Model file for the job. Use its own axes, mm. Face numbers are marked on the shaded views. A direction names the side the tool comes from. Round coordinates to 2 decimals unless told otherwise and drop trailing zeros. One line per item, written item: value.
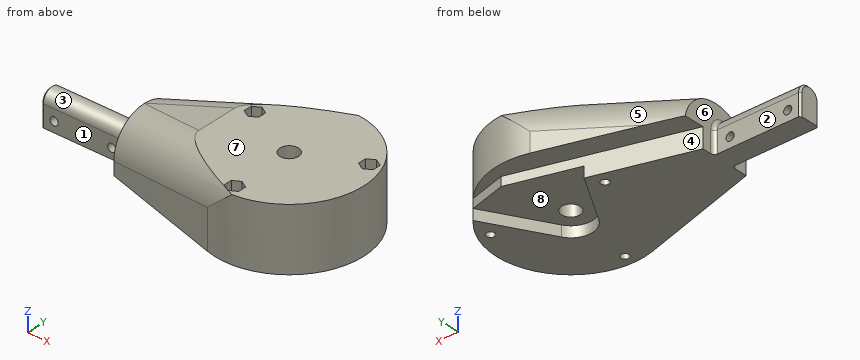
from build123d import *

# Parameters (mm, degrees)
RESSALTO_EXTRUS_O1_DEPTH = 35
CHANFRO1_SIZE            = 40
CHANFRO1_SIZE2           = 8.502262467
FILETE2_R                = 20
CORTE_EXTRUS_O2_DEPTH    = 6
CORTE_EXTRUS_O3_DEPTH    = 11
CHANFRO2_SIZE            = 10
RESSALTO_EXTRUS_O2_DEPTH = 48
CHANFRO3_SIZE            = 1
FILETE3_R                = 2
ESBO_O9_R                = 2.25
CORTE_EXTRUS_O4_DEPTH    = 342.284989024
ESBO_O10_R               = 5.15
CORTE_EXTRUS_O5_DEPTH    = 367.917618461
CORTE_EXTRUS_O7_DEPTH    = 10
ESBO_O13_R               = 2.25
CORTE_EXTRUS_O8_DEPTH    = 367.09908322


with BuildPart() as part:
    # Esboço1 → Ressalto-extrusão1 (new body)
    with BuildSketch(Plane.XY):
        with BuildLine():
            Line((-288.88140452, 80), (-220.127979697, 60.449355997))
            ThreePointArc((-220.127979697, 60.449355997), (-167.76280904, 100), (-220.127979697, 139.550644003))
            Line((-220.127979697, 139.550644003), (-288.88140452, 119.635273108))
            Line((-288.88140452, 119.635273108), (-288.88140452, 80))
        make_face()
    extrude(amount=RESSALTO_EXTRUS_O1_DEPTH)

    # Chanfro1
    chanfro1_edges = [part.edges().sort_by_distance(p)[0] for p in [
        (-288.88140452, 99.817636554, 35),
    ]]
    chanfro1_side = [part.faces().sort_by_distance(p)[0] for p in [
        (-225.798931966, 99.956743446, 35),
    ]]
    chamfer(chanfro1_edges, length=CHANFRO1_SIZE, length2=CHANFRO1_SIZE2, reference=chanfro1_side[0])

    # Filete2
    # the kernel refuses this fillet: 20 mm, written as the material it takes off along each edge
    with BuildSketch(Plane(origin=(-115.658970437, 169.81152296, 63.317302526), x_dir=(0.19213899287120792, 0.055655690116350805, -0.9797882687479528), z_dir=(-0.9411018224853822, -0.27260302876307696, -0.2000373675688854))) as filete2_piece_1:
        with BuildLine():
            CenterArc((FILETE2_R * 0.943733759019, FILETE2_R), FILETE2_R, 183.31621355, 86.68378645)
            Line((-FILETE2_R * 0.054591728164, FILETE2_R * 0.942153464743), (0, 0))
            Line((0, 0), (FILETE2_R * 0.943733759019, 0))
        make_face()
    extrude(amount=231.2501229, mode=Mode.SUBTRACT)
    with BuildSketch(Plane(origin=(-115.347800558, 30.654185994, 63.383443726), x_dir=(0.2621163849534368, 0.9634266390424966, 0.05571455754307817), z_dir=(-0.9423734554624519, 0.2679722209171675, -0.2003076615021976))) as filete2_piece_2:
        with BuildLine():
            CenterArc((FILETE2_R * 0.9446616108, FILETE2_R), FILETE2_R, 183.260002361, 86.739997639)
            Line((-FILETE2_R * 0.0537201474496, FILETE2_R * 0.943132919942), (0, 0))
            Line((0, 0), (FILETE2_R * 0.9446616108, 0))
        make_face()
    extrude(amount=231.378339467, mode=Mode.SUBTRACT)

    # Esboço6 → Corte-extrusão2 (cut)
    with BuildSketch(Plane(origin=(0, 0, 0), x_dir=(-1, 0, 0), z_dir=(0, 0, -1))):
        with BuildLine():
            Line((219.273709365, 94), (245.2234198, 138.946216915))
            Line((245.2234198, 138.946216915), (172.539389239, 138.946216915))
            Line((172.539389239, 138.946216915), (198.489099675, 94))
            ThreePointArc((198.489099675, 94), (208.88140452, 88), (219.273709365, 94))
        make_face()
    extrude(amount=-CORTE_EXTRUS_O2_DEPTH, mode=Mode.SUBTRACT)

    # Esboço7 → Corte-extrusão3 (cut)
    with BuildSketch(Plane(origin=(0, 0, 0), x_dir=(-1, 0, 0), z_dir=(0, 0, -1))):
        Polygon((179.171530951, 139.11313265), (295.618088129, 106.000524942), (295.618088129, 136.423544796), (188.948158446, 165.308096575), align=None)
    extrude(amount=-CORTE_EXTRUS_O3_DEPTH, mode=Mode.SUBTRACT)

    # Chanfro2
    # the kernel refuses this chamfer: 22.612495948, 10 mm, written as the material it takes off along each edge
    with BuildSketch(Plane(origin=(-189.392572811, 136.206689062, 11), x_dir=(0.7913619734687217, -0.6113478771924299, 0), z_dir=(0, 0, -1))) as chanfro2_piece_1:
        with BuildLine():
            Line((13.424324353, 0), (-CHANFRO2_SIZE * 0.593972278099, CHANFRO2_SIZE * 0.804485508167))
            Line((-CHANFRO2_SIZE * 0.593972278099, CHANFRO2_SIZE * 0.804485508167), (0, 0))
            ThreePointArc((0, 0), (7.133656498, -0.549382314), (13.424324353, 0))
        make_face()
    extrude(amount=40.659571502, mode=Mode.SUBTRACT)

    # Esboço8 → Ressalto-extrusão2 (add)
    with BuildSketch(Plane.ZY.offset(288.88140452)):
        with BuildLine():
            Line((0, 100.85), (12, 100.85))
            ThreePointArc((12, 100.85), (17.85, 95), (12, 89.15))
            Line((12, 89.15), (0, 89.15))
            Line((0, 89.15), (0, 100.85))
        make_face()
    extrude(amount=RESSALTO_EXTRUS_O2_DEPTH)

    # Chanfro3
    chanfro3_edges = [part.edges().sort_by_distance(p)[0] for p in [
        (-336.88140452, 89.15, 6),
        (-336.88140452, 95, 17.85),
        (-336.88140452, 100.85, 6),
    ]]
    chamfer(chanfro3_edges, length=CHANFRO3_SIZE)

    # Filete3
    filete3_edges = [part.edges().sort_by_distance(p)[0] for p in [
        (-288.88140452, 89.15, 6),
        (-288.88140452, 95, 17.85),
        (-288.88140452, 100.85, 6),
    ]]
    fillet(filete3_edges, radius=FILETE3_R)

    # Esboço9 → Corte-extrusão4 (cut, through all)
    with BuildSketch(Plane(origin=(0, 100.85, 0), x_dir=(1, 0, 0), z_dir=(0, 1, 0))):
        with Locations(Location((-329.846296891, -5.75110431, 0), (0, 0, 270))):
            Circle(ESBO_O9_R)
        with Locations(Location((-297.910035946, -5.75110431, 0), (0, 0, 270))):
            Circle(ESBO_O9_R)
    extrude(amount=-CORTE_EXTRUS_O4_DEPTH, mode=Mode.SUBTRACT)

    # Esboço10 → Corte-extrusão5 (cut, through all)
    with BuildSketch(Plane(origin=(0, 0, 0), x_dir=(-1, 0, 0), z_dir=(0, 0, -1))):
        with Locations((208.88140452, 100)):
            Circle(ESBO_O10_R)
    extrude(amount=-CORTE_EXTRUS_O5_DEPTH, mode=Mode.SUBTRACT)

    # Esboço12 → Corte-extrusão7 (cut)
    with BuildSketch(Plane.XY.offset(35)):
        Polygon((-240.599798192, 119.415541755), (-244.599798192, 117.106140678), (-244.599798192, 112.487338525), (-240.599798192, 110.177937448), (-236.599798192, 112.487338525), (-236.599798192, 117.106140678), align=None)
        Polygon((-208.88140452, 69.618802154), (-212.88140452, 67.309401077), (-212.88140452, 62.690598923), (-208.88140452, 60.381197846), (-204.88140452, 62.690598923), (-204.88140452, 67.309401077), align=None)
        Polygon((-177.163010847, 119.415541755), (-181.163010847, 117.106140678), (-181.163010847, 112.487338525), (-177.163010847, 110.177937448), (-173.163010847, 112.487338525), (-173.163010847, 117.106140678), align=None)
    extrude(amount=-CORTE_EXTRUS_O7_DEPTH, mode=Mode.SUBTRACT)

    # Esboço13 → Corte-extrusão8 (cut, through all)
    with BuildSketch(Plane.XY.offset(25)):
        with Locations((-177.163010847, 114.796739602)):
            Circle(ESBO_O13_R)
        with Locations((-208.88140452, 65)):
            Circle(ESBO_O13_R)
        with Locations((-240.599798192, 114.796739602)):
            Circle(ESBO_O13_R)
    extrude(amount=-CORTE_EXTRUS_O8_DEPTH, mode=Mode.SUBTRACT)


solid = part.part
1. Wall check: probe 1 along Z at (x, y) = (-248.5, 86); probe 2 along Y at (x, z) = (-314, 10); probe 3 along X at (y, z) = (102.5, 23). Give the ranges that are in metal, low to high. Write a range as [from, to].
Report:
probe 1: [0, 34.97]
probe 2: [89.15, 100.85]
probe 3: [-288.88, -213.38], [-204.38, -167.84]
2. Tool access for the marked faces 1, 2, 3, 4 and 5: list every direction of +Z, -Z, +X, -X, +Y, -Y with a clear straight run to the whole face (end or side of a thin tool).
Report:
face 1: +Z, -Z, -X, -Y
face 2: +Z, -Z, -X, +Y
face 3: +Z, -X
face 4: -Z, -X, +Y
face 5: +Z, -X, +Y
3. Band-saw the part on A-A on z = 29. State how many separate pieces and enclosed holes the cut face has, plus the area to 3 significant figures.
Report:
separate pieces: 1
enclosed holes: 4
area: 6,160 mm²
4. Drop flat-ended pins along their axis: pin 1 (7 mm diameter, centred on x = -297.91, z = 5.75, fed in from +Y); pin 2 (13 mm diameter, centred on x = -319, z = 5, fed in from -Y); pin 3 (5 mm diameter, centred on y = 64, z = 30.5, fed in from +X). Give the stop position or say it passes through.
Report:
pin 1: y = 100.85
pin 2: y = 89.15
pin 3: x = -185.04
5. Mould opens along X. For the marked faces 6, 7 and 8 say: released by +X, released by -X, zero draft, split by the parting line, or undercut.
Report:
face 6: released by -X
face 7: zero draft
face 8: undercut
